from build123d import *

# Parameters (mm, degrees)
SKETCH_1_R      = 1.5
EXTRUDE_1_DEPTH = 3.5
SKETCH_2_R      = 2.75
SKETCH_2_R_2    = 1.5
EXTRUDE_2_DEPTH = 0.5
FILLET_4_R      = 0.2
FILLET_5_R      = 0.2


with BuildPart() as part:
    # 草图1 → 凸台-拉伸1 (new body)
    with BuildSketch(Plane.XY):
        Polygon((3.175426481, 0), (1.58771324, 2.75), (-1.58771324, 2.75), (-3.175426481, 0), (-1.58771324, -2.75), (1.58771324, -2.75), align=None)
        Circle(SKETCH_1_R, mode=Mode.SUBTRACT)
    extrude(amount=EXTRUDE_1_DEPTH)

    # 草图2 → 凸台-拉伸2 (add)
    with BuildSketch(Plane.XY.offset(3.5)):
        Circle(SKETCH_2_R)
        Circle(SKETCH_2_R_2, mode=Mode.SUBTRACT)
    extrude(amount=EXTRUDE_2_DEPTH)

    # 圆角4
    fillet_4_edges = [part.edges().sort_by_distance(p)[0] for p in [
        (-2.75, 0, 4),
    ]]
    fillet(fillet_4_edges, radius=FILLET_4_R)

    # 圆角5
    fillet_5_edges = [part.edges().sort_by_distance(p)[0] for p in [
        (0, -2.75, 0),
        (-2.38156986, -1.375, 0),
        (-2.38156986, 1.375, 0),
        (0, 2.75, 0),
        (2.38156986, 1.375, 0),
        (2.38156986, -1.375, 0),
    ]]
    fillet(fillet_5_edges, radius=FILLET_5_R)


solid = part.part
The listing builds one solid part. Answer for the finished solid, in the listing's coordinates (mm). A direction names the side the tool comes from. Round coordinates to 2 decimals unless told otherwise and drop trailing zeros. Write each question's results on one line, items separated by ' | '. Start each with the question number.
Item 1: Given pin 1 Ø1 at (y, z) = (-1, 1.5) entering from -X, flat-ended and moving along its own axis, determine where the tip first touches the part or whether it passes through.
Item 2: Straight lines are drawn through the part: probe 1 along Y at (x, z) = (0, 1.95); probe 2 along X at (y, z) = (-1, 2.3); probe 3 along Y at (x, z) = (1.25, 0.9). For each, find the intervals that lie inside material, in ascending order.
Item 3: Which of the six approach directions +Z, -Z, +X, -X, +Y, -Y give full straight-line access (tool end or side, diameter ignored) to faces 5 (the flat face through (-1.5, 2.5, 3.5)), 6 (the flat face through (-1.5, -2.5, 3.5)), 7 (the flat face through (1.45, -2.52, 3.5))?
Item 4: The mould has two halves that part along Y. Classify faces 1 (the cylindrical face through (-1.5, 0.07, 1.97)), 2 (the cylindrical face through (-2.32, -1.37, 0.06)), 3 (the flat face through (0, 2.75, 2)), 4 (the flat face through (0, -2, 4)): +Y half, -Y half, draft (parallel to the pull), parting line (faces both ways), or undercut.
Answer block:
1) pin 1: stops at x = -2.89
2) probe 1: y = -2.75 to -1.5, 1.5 to 2.75 | probe 2: x = -2.6 to -1.12, 1.12 to 2.6 | probe 3: y = -2.75 to -0.83, 0.83 to 2.75
3) face 5: +Z, -X, +Y | face 6: +Z, -X, -Y | face 7: +Z, +X, -Y
4) face 1: undercut | face 2: -Y half | face 3: +Y half | face 4: draft
